```python
from build123d import *

# Parameters (mm, degrees)
SKETCH1_R           = 4.699
BOSS_EXTRUDE1_DEPTH = 2.7178
SKETCH2_R           = 2.159
BOSS_EXTRUDE2_DEPTH = 38.1
SKETCH3_W           = 4.064
SKETCH3_H           = 4.064
CUT_EXTRUDE1_DEPTH  = 2.286
FILLET2_R           = 0.254


with BuildPart() as part:
    # Sketch1 → Boss-Extrude1 (new body)
    with BuildSketch(Plane(origin=(0, 0, 0), x_dir=(1, 0, 0), z_dir=(0, 1, 0))):
        with Locations(Location((0, 0, 0), (0, 0, 270))):
            Circle(SKETCH1_R)
    extrude(amount=-BOSS_EXTRUDE1_DEPTH)

    # Sketch2 → Boss-Extrude2 (add)
    with BuildSketch(Plane(origin=(0, 0, 0), x_dir=(1, 0, 0), z_dir=(0, 1, 0))):
        with Locations(Location((0, 0, 0), (0, 0, 270))):
            Circle(SKETCH2_R)
    extrude(amount=-BOSS_EXTRUDE2_DEPTH)

    # Sketch3 → Cut-Extrude1 (cut)
    with BuildSketch(Plane(origin=(0, 0, 0), x_dir=(1, 0, 0), z_dir=(0, 1, 0))):
        Rectangle(SKETCH3_W, SKETCH3_H)
    extrude(amount=-CUT_EXTRUDE1_DEPTH, mode=Mode.SUBTRACT)

    # Fillet2
    fillet2_edges = [part.edges().sort_by_distance(p)[0] for p in [
        (0, 0, -4.699),
        (0, -2.7178, -4.699),
    ]]
    fillet(fillet2_edges, radius=FILLET2_R)


solid = part.part
```
Input: part model. Units: mm. Frame: model coordinates. A direction names the side the tool comes from. Coordinates: 2 decimals unless noted, no trailing zeros. Loops run counter-clockwise (first coordinate to the right, second up) from the corner with the lowest first, then second, coordinate; pieces in that order, holes last. Notation, with made-up numbers: M 75.25,-14.75 L 102.25,-14.75 A20 ccw 102.25,-0.75 Z; hole C -31.5,-12.75 d9. An arc over 180 degrees is marked long. Use a Markdown table: item, result. Add a question column.
1) Draft query along X for faces 3 (the flat face through (0, -1, -2.032)), 4 (the flat face through (0, -38.1, 0)), 5 (the cylindrical face through (4.66, -1.34, -0.61)). Return one class per face: +X half, -X half, draft (parallel to the pull), parting line (faces both ways), or undercut.
2) Section B-B, the plane x = 0. Return the cut outline in (y, z) (3 decimals), plus the area to 3 significant figures.
3) Line query: L1, parallel to Y at x = -2.75, z = 3.25; L2, parallel to Y at x = 0.5, z = 1; L3, parallel to Z at x = -0.75, y = -27. Output: solid intervals per line, ascending. Write a range as from..to.
4) Section A-A, the plane z = 0. Return the cut outline in (x, y) (3 decimals), plus the area to 3 significant figures.
5) Section C-C, the plane y = -9. Return the cut outline in (x, z), plus the area to 3 significant figures.
6) Set-up query: faces 1 (the cylindrical face through (2.14, -20.16, -0.28)), 2 (the flat face through (0, -2.286, 0)). Return all of +Z, -Z, +X, -X, +Y, -Y with unobstructed straight access to the full face (end or side cutting, diameter ignored); none if empty.
7) Pin query (flat end, axial travel): P1, Ø0.7, axis at x = -0.5, y = -1.5, coming from the -Z side; P2, Ø1.5, axis at x = 2, y = -11.5, coming from the -Z side; P3, Ø4, axis at x = 1, y = -27.5, coming from the +Z side. Return the tip coordinate at first contact, or that it passes through.
Answer below:
| question | item | result |
|---|---|---|
| 1 | face 3 | undercut |
| 1 | face 4 | draft |
| 1 | face 5 | parting line |
| 2 | outline | M -38.1,-2.159 L -2.718,-2.159 L -2.718,-4.445 A0.254 ccw -2.464,-4.699 L -0.254,-4.699 A0.254 ccw 0,-4.445 L 0,-2.032 L -2.286,-2.032 L -2.286,2.032 L 0,2.032 L 0,4.445 A0.254 ccw -0.254,4.699 L -2.464,4.699 A0.254 ccw -2.718,4.445 L -2.718,2.159 L -38.1,2.159 Z |
| 2 | area | 169 mm2 |
| 3 | L1 | -2.72..0 |
| 3 | L2 | -38.1..-2.29 |
| 3 | L3 | -2.02..2.02 |
| 4 | outline | M -4.699,-2.464 A0.254 ccw -4.445,-2.718 L -2.159,-2.718 L -2.159,-38.1 L 2.159,-38.1 L 2.159,-2.718 L 4.445,-2.718 A0.254 ccw 4.699,-2.464 L 4.699,-0.254 A0.254 ccw 4.445,0 L 2.032,0 L 2.032,-2.286 L -2.032,-2.286 L -2.032,0 L -4.445,0 A0.254 ccw -4.699,-0.254 Z |
| 4 | area | 169 mm2 |
| 5 | outline | C 0,0 d4.32 |
| 5 | area | 14.6 mm2 |
| 6 | face 1 | -Y |
| 6 | face 2 | +Y |
| 7 | P1 | z = -4.7 |
| 7 | P2 | z = -1.76 |
| 7 | P3 | z = 2.16 |
